from build123d import *

# Parameters (mm, degrees)
SKETCH_W         = 74
SKETCH_H         = 11.5
EXTRUDE002_DEPTH = 10
SKETCH007_R      = 3.7
EXTRUDE001_DEPTH = 11.5
SKETCH006_R      = 5.3
SKETCH006_R_2    = 2
EXTRUDE_DEPTH    = 9
BOX001_W         = 115.8
BOX001_H         = 106
BOX001_DEPTH     = 1.5


with BuildPart() as extrude002:
    # Sketch → Extrude002 (new body)
    with BuildSketch(Plane.XY.offset(3.5)):
        with Locations((-9, -26.75)):
            Rectangle(SKETCH_W, SKETCH_H)
    extrude(amount=-EXTRUDE002_DEPTH)


with BuildPart() as extrude001:
    # Sketch007 → Extrude001 (new body)
    with BuildSketch(Plane.XY.offset(2)):
        with Locations((-50.25, -47.25)):
            Circle(SKETCH007_R)
        with Locations((50.25, 47.25)):
            Circle(SKETCH007_R)
        with Locations((-50.25, 47.25)):
            Circle(SKETCH007_R)
        with Locations((25.25, -42.25)):
            Circle(SKETCH007_R)
    extrude(amount=-EXTRUDE001_DEPTH)


with BuildPart() as extrude001_1:
    # Extrude001 placement: moved
    add(extrude001.part.moved(Location((0, 0, 4))))


with BuildPart() as extrude_mount_columns:
    # Sketch006 → Extrude (new body)
    with BuildSketch(Plane.XY.offset(2)):
        with Locations((-50.25, -47.25)):
            Circle(SKETCH006_R)
        with Locations((-50.25, -47.25)):
            Circle(SKETCH006_R_2, mode=Mode.SUBTRACT)
        with Locations((50.25, 47.25)):
            Circle(SKETCH006_R)
        with Locations((50.25, 47.25)):
            Circle(SKETCH006_R_2, mode=Mode.SUBTRACT)
        with Locations((-50.25, 47.25)):
            Circle(SKETCH006_R)
        with Locations((-50.25, 47.25)):
            Circle(SKETCH006_R_2, mode=Mode.SUBTRACT)
        with Locations((25.25, -42.25)):
            Circle(SKETCH006_R)
        with Locations((25.25, -42.25)):
            Circle(SKETCH006_R_2, mode=Mode.SUBTRACT)
    extrude(amount=-EXTRUDE_DEPTH)


with BuildPart() as cut001:
    # Box001 → Box001 (new body)
    with BuildSketch(Plane(origin=(-60, -53, 2), x_dir=(1, 0, 0), z_dir=(0, 0, 1))):
        with Locations((57.9, 53)):
            Rectangle(BOX001_W, BOX001_H)
    extrude(amount=BOX001_DEPTH)

    # Fusion: union Extrude Mount Columns
    add(extrude_mount_columns.part)

    # Cut: cut Extrude001
    add(extrude001_1.part, mode=Mode.SUBTRACT)

    # Cut001: cut Extrude002
    add(extrude002.part, mode=Mode.SUBTRACT)


solid = cut001.part
Geometry: final body of the model. Coordinates: model frame, mm. A direction names the side the tool comes from. Round coordinates to 2 decimals unless told otherwise and drop trailing zeros. Loops run counter-clockwise (first coordinate to the right, second up) from the corner with the lowest first, then second, coordinate; pieces in that order, holes last. Notation, with made-up numbers: (46, 32.25) -> (87, 32.25) arc R22 ccw to (87, 38.25) -> close; hole circle Ø7 at (-35, -28). An arc over 180 degrees is marked (long way). One line per question, with ' | ' between items. Start each with the question number.
1. Set-up query: faces 4 (the face through (-3, 1, 2)), 5 (the face through (50, 45, -7)), 6 (the face through (47.52, 49.75, -0.94)). Return all of +Z, -Z, +X, -X, +Y, -Y with unobstructed straight access to the full face (end or side cutting, diameter ignored); none if empty.
2. Section C-C on x = 50.25. Output: boundary loops of the cut face in (y, z).
3. Section B-B on z = -2.25. Output: boundary loops of the cut face in (x, y), and give its area (3 significant figures).
4. Section A-A on y = 47.25. Output: boundary loops of the cut face in (x, z), and give its area (3 significant figures).
5. Line query: line 1 along Y through (x, z) = (50.25, -2.5); line 2 along Y through (x, z) = (-50.25, -6.45); line 3 along X through (y, z) = (-47.5, 2.5). Output: solid intervals per line, ascending. Write a range as [from, to].
6. Contact query for flat-ended pins moving along their axis: pin 1 (8 mm diameter, centred on x = -50.5, y = -49, fed in from +Z); pin 2 (1 mm diameter, centred on x = 43.5, y = 20.5, fed in from -Z); pin 3 (3.5 mm diameter, centred on x = 50.25, y = 47.25, fed in from +Z) (3 decimals); pin 4 (3.5 mm diameter, centred on x = 25.5, y = -43.5, fed in from +Z). Output: stop coordinate, or through.
7. Mould query, pull axis Y, two halves, no side actions, for faces 1 (the face through (28, -42, -7)), 2 (the face through (49.101, 42.076, -2.437)), 3 (the face through (-51.399, -52.424, -2.437)). Classes: pulls with the +Y half, pulls with the -Y half, needs draft (parallel to the pull), parting line crosses it, or undercut.
8. Section D-D on x = 25.25. Output: boundary loops of the cut face in (y, z).
Returned:
1) face 4: -Z | face 5: -Z, +X, -X, +Y, -Y | face 6: +Z
2) outline: (-53, 2) -> (41.95, 2) -> (41.95, -7) -> (45.25, -7) -> (45.25, -5.5) -> (43.55, -5.5) -> (43.55, 3.5) -> (-53, 3.5) -> close; (49.25, -7) -> (52.55, -7) -> (52.55, 2) -> (53, 2) -> (53, 3.5) -> (50.95, 3.5) -> (50.95, -5.5) -> (49.25, -5.5) -> close
3) outline: circle Ø10.6 at (-50.25, -47.25); circle Ø10.6 at (-50.25, 47.25); circle Ø10.6 at (25.25, -42.25); circle Ø10.6 at (50.25, 47.25); hole circle Ø7.4 at (-50.25, -47.25); hole circle Ø7.4 at (-50.25, 47.25); hole circle Ø7.4 at (25.25, -42.25); hole circle Ø7.4 at (50.25, 47.25) | area: 181 mm2
4) outline: (-60, 2) -> (-55.55, 2) -> (-55.55, -7) -> (-52.25, -7) -> (-52.25, -5.5) -> (-53.95, -5.5) -> (-53.95, 3.5) -> (-60, 3.5) -> close; (-48.25, -7) -> (-44.95, -7) -> (-44.95, 2) -> (44.95, 2) -> (44.95, -7) -> (48.25, -7) -> (48.25, -5.5) -> (46.55, -5.5) -> (46.55, 3.5) -> (-46.55, 3.5) -> (-46.55, -5.5) -> (-48.25, -5.5) -> close; (52.25, -7) -> (55.55, -7) -> (55.55, 2) -> (55.8, 2) -> (55.8, 3.5) -> (53.95, 3.5) -> (53.95, -5.5) -> (52.25, -5.5) -> close | area: 219 mm2
5) line 1: y = [41.95, 43.55], [50.95, 52.55] | line 2: y = [-52.55, -49.25], [-45.25, -41.95], [41.95, 45.25], [49.25, 52.55] | line 3: x = [-60, -53.94], [-46.56, 55.8]
6) pin 1: stops at z = 3.5 | pin 2: stops at z = 2 | pin 3: passes through | pin 4: stops at z = -5.5
7) face 1: needs draft | face 2: parting line crosses it | face 3: undercut
8) outline: (-53, 2) -> (-47.55, 2) -> (-47.55, -7) -> (-44.25, -7) -> (-44.25, -5.5) -> (-45.95, -5.5) -> (-45.95, 3.5) -> (-53, 3.5) -> close; (-40.25, -7) -> (-36.95, -7) -> (-36.95, 2) -> (-32.5, 2) -> (-32.5, 3.5) -> (-38.55, 3.5) -> (-38.55, -5.5) -> (-40.25, -5.5) -> close; (-21, 2) -> (53, 2) -> (53, 3.5) -> (-21, 3.5) -> close
